Verification items for the finished model (mm, model axes). Face numbers are marked on the shaded views. A direction names the side the tool comes from. Give positions to 0.01 mm unless a question says otherwise; leave off trailing zeros. Order: outer loops, then holes, each group sorted by start corner. A loop starts at its lowest first (then second) coordinate and runs counter-clockwise, first axis right, second up. Notation, with made-up numbers: M -13.75,75 L 23.25,75 A22 ccw 23.25,98 Z; hole C 37,45.25 d6. An arc over 180 degrees is marked long. Answer as a JSON object with one key per item and string values.
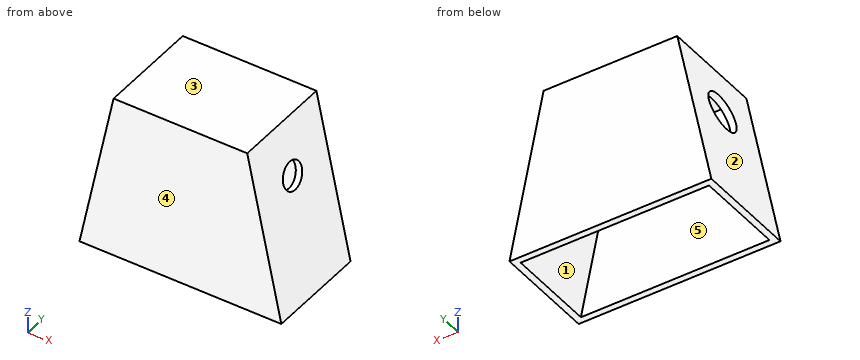
```python
from build123d import *

# Parameters (mm, degrees)
F1_DEPTH = 7.84
F3_T     = -0.5
F2_R     = 1.0501143569
F4_DEPTH = 0.5
F5_R     = 1.5374067345
F6_DEPTH = 0.5


with BuildPart() as f1:
    # F0 (on Front) → F1 (new body)
    with BuildSketch(Plane.XZ):
        Polygon((2.6, 12.5025157468), (0, 0), (15.4, 0), (12.8, 12.5025157468), align=None)
    extrude(amount=F1_DEPTH)

    # F3
    f3_openings = [f1.faces().sort_by_distance(p)[0] for p in [
        (7.7, -3.92, 0),
    ]]
    offset(amount=F3_T, openings=f3_openings)

    # F2 (on face) → F4 (cut, through all)
    with BuildSketch(Plane(origin=(14.7616106661, 0, 3.069797192), x_dir=(0, 1, 0), z_dir=(0.9790536998, 0, 0.2036021926))):
        with Locations((-3.92, 5.6268600747)):
            Circle(F2_R)
    extrude(amount=-F4_DEPTH, mode=Mode.SUBTRACT)

    # F5 (on face) → F6 (cut, through all)
    with BuildSketch(Plane(origin=(0, 0, 0), x_dir=(0, -1, 0), z_dir=(-0.9790536998, 0, 0.2036021926))):
        with Locations((3.92, 8.7754800916)):
            Circle(F5_R)
    extrude(amount=-F6_DEPTH, mode=Mode.SUBTRACT)


solid = f1.part
```
Q1. Section check D-D on y = -1. Record the cut outline in (x, z).
Resolved:
{"outline": "M 0,0 L 0.51,0 L 3.01,12 L 12.39,12 L 14.89,0 L 15.4,0 L 12.8,12.5 L 2.6,12.5 Z"}
Q2. Tool access check on the marked faces 4 and 5. Record the directions out of +Z, -Z, +X, -X, +Y, -Y that give a thin tool (end or side, any length) a straight path to the whole face; none if there is none.
Resolved:
{"face 4": "+Z, -Z, +X, -X, -Y", "face 5": "-Z"}
Q3. Release check for a two-part mould opening along X. For the marked faces 1, 2 and 3 record: +X half, -X half, draft (parallel to the pull), parting line (faces both ways), or undercut.
Resolved:
{"face 1": "undercut", "face 2": "-X half", "face 3": "draft"}
Q4. Gauge pin test, flat end, axial feed: pin 1 Ø2 at (y, z) = (-6, 9.5) entering from -X. Record the tip position at first contact, or that the pin passes through.
Resolved:
{"pin 1": "stops at x = 1.77"}
Q5. Section check C-C on x = 7.5. Record the cut outline in (y, z).
Resolved:
{"outline": "M -7.84,0 L -7.34,0 L -7.34,12 L -0.5,12 L -0.5,0 L 0,0 L 0,12.5 L -7.84,12.5 Z"}
Q6. Section check B-B on z = 1. Record the cut outline in (x, y).
Resolved:
{"outline": "M 0.21,-7.84 L 15.19,-7.84 L 15.19,0 L 0.21,0 Z; hole M 0.72,-7.34 L 14.68,-7.34 L 14.68,-0.5 L 0.72,-0.5 Z"}
Q7. Material ranges on L1, parallel to Y at x = 4, z = 8.25; L2, parallel to X at y = -7, z = 3.5; L3, parallel to Z at x = 8.5, y = -6, recorded low to high.
Resolved:
{"L1": "y = -7.84 to -7.34, -0.5 to 0", "L2": "x = 0.73 to 1.24, 14.16 to 14.67", "L3": "z = 12 to 12.5"}
Q8. Section check A-A on y = -4.25. Record the cut outline in (x, z).
Resolved:
{"outline": "M 0,0 L 0.51,0 L 1.97,7.02 L 1.48,7.12 Z; M 2.09,10.06 L 2.58,9.96 L 3.01,12 L 12.39,12 L 12.92,9.45 L 13.41,9.55 L 12.8,12.5 L 2.6,12.5 Z; M 13.33,7.5 L 14.89,0 L 15.4,0 L 13.82,7.6 Z"}
